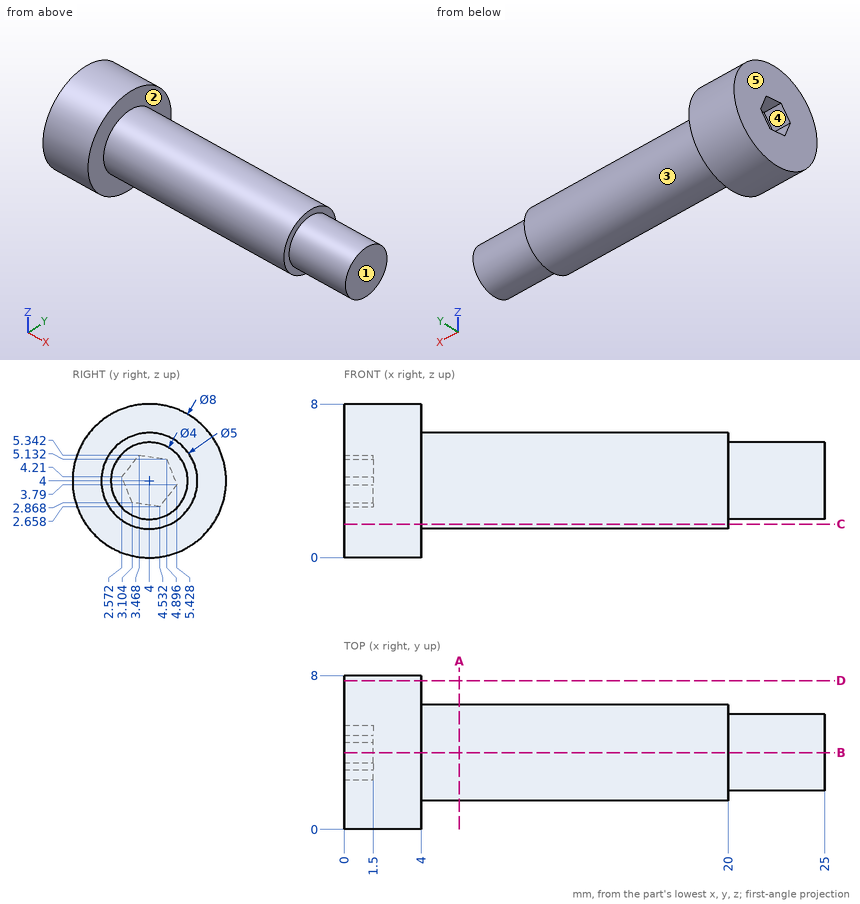
Geometry: see drawing. Coordinates: mm, zero at the bounding-box minimum. A direction names the side the tool comes from. Give positions to 0.01 mm unless a question says otherwise; leave off trailing zeros. Write each loop counter-clockwise with the first axis right and the second up, starting at its lowest first coordinate (ties: lowest second). Pieces come first, ordered by that corner, then holes. Notation, with made-up numbers: M 81,2 L 117,2 A28 ccw 117,21 Z; hole C 9,70 d3. An arc over 180 degrees is marked long. Answer in a Markdown table with one row per item. Add a question column.
(1) Section D-D on y = 7.75. Return loops of the section in (x, z).
(2) Ray query, line 1 (X direction, y = 1, z = 5); line 2 (X direction, y = 4, z = 3); line 3 (Y direction, x = 11.75, z = 3). Return the intervals inside material, ascending.
(3) Reachability of the marked faces 1 and 2 from +Z, -Z, +X, -X, +Y, -Y: full face, straight path, thin tool, end or side. Return the list, or none.
(4) First-contact query: pin 1 (1.5 mm diameter, centred on y = 5.5, z = 6.5, fed in from -X); pin 2 (1.5 mm diameter, centred on x = 16, y = 2.5, fed in from +Z) (1 decimal); pin 3 (0.8 mm diameter, centred on y = 3.5, z = 4, fed in from -X); pin 4 (4 mm diameter, centred on x = 16, y = 7, fed in from -Z). Flat tips, straight axial feed; report the tip coordinate or a pass-through.
(5) Section C-C on z = 1.75. Return loops of the section in (x, y).
(6) Section A-A on x = 6. Return loops of the section in (y, z).
(7) Mould query, pull axis Y, two halves, no side actions, for the marked faces 3, 4 and 5. Classes: +Y half, -Y half, draft (parallel to the pull), parting line (faces both ways), or undercut.
(8) Section B-B on y = 4. Return loops of the section in (x, z), and give its area (3 significant figures).
Result set:
| question | item | result |
|---|---|---|
| 1 | outline | M 0,2.61 L 4,2.61 L 4,5.39 L 0,5.39 Z |
| 2 | line 1 | x = 0 to 4 |
| 2 | line 2 | x = 1.5 to 25 |
| 2 | line 3 | y = 1.71 to 6.29 |
| 3 | face 1 | +Z, -Z, +X, +Y, -Y |
| 3 | face 2 | +X |
| 4 | pin 1 | stops at x = 0 |
| 4 | pin 2 | stops at z = 6.4 |
| 4 | pin 3 | stops at x = 1.5 |
| 4 | pin 4 | stops at z = 1.71 |
| 5 | outline | M 0,0.69 L 4,0.69 L 4,2.91 L 20,2.91 L 20,5.09 L 4,5.09 L 4,7.31 L 0,7.31 Z |
| 6 | outline | C 4,4 d5 |
| 7 | face 3 | parting line |
| 7 | face 4 | undercut |
| 7 | face 5 | draft |
| 8 | outline | M 0,0 L 4,0 L 4,1.5 L 20,1.5 L 20,2 L 25,2 L 25,6 L 20,6 L 20,6.5 L 4,6.5 L 4,8 L 0,8 L 0,5.26 L 1.5,5.26 L 1.5,2.74 L 0,2.74 Z |
| 8 | area | 128 mm^2 |
